For this review, take the finished solid that the model builds, in its own axes (mm). Coordinates: 2 decimals unless noted, no trailing zeros. Write each loop counter-clockwise with the first axis right and the second up, starting at its lowest first coordinate (ties: lowest second). Pieces come first, ordered by that corner, then holes.
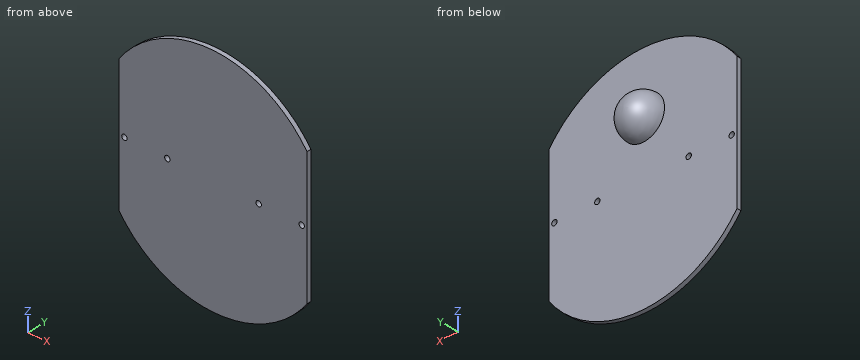
Autodesk Inventor part; units mm, degrees
ref_plane "YZ Plane" through (0, 0, 0) normal (1, 0, 0) x (0, 1, 0)
ref_plane "XZ Plane" through (0, 0, 0) normal (0, 1, 0) x (-1, 0, 0)
ref_plane "XY Plane" through (0, 0, 0) normal (0, 0, 1) x (1, 0, 0)
sketch "Sketch1" plane through (0, 0, 0) normal (0, 1, 0) x (-1, 0, 0)
  line L0 (44.45, 31.7246) -> (44.45, -31.7246)
  line L1 (-44.45, -31.7246) -> (-44.45, 31.7246)
  arc A0 (-44.45, -31.7246) -> (44.45, -31.7246) centre (0, 0) ccw
  arc A1 (44.45, 31.7246) -> (-44.45, 31.7246) centre (0, 0) ccw
  line L2 (44.45, 0) -> (41.91, 0)
  circle A2 centre (41.91, 0) radius 1.27
  line L3 (41.91, 0) -> (21.59, 0)
  circle A3 centre (21.59, 0) radius 1.27
  line L4 (0, -54.61) -> (0, 54.61)
  circle A4 centre (-41.91, 0) radius 1.27
  circle A5 centre (-21.59, 0) radius 1.27
  dimension "d3" = 88.9
  dimension "d4" = 2.54
  dimension "d5" = 2.54
  dimension "d6" = 20.32
  dimension "d7" = 2.54
extrude "Extrusion1" add sketch "Sketch1" along normal blind 2.032
sketch "Sketch2" plane through (0, 2.032, 0) normal (0, 1, 0) x (1, 0, 0)
  circle A0 centre (0, -25.3797) radius 10.16
  point P0 (0, 0)
  dimension "d10" = 20.32
extrude "Extrusion2" add sketch "Sketch2" along normal blind 10.16
fillet "Fillet1" radius 10.16 1 edges at (-10.16, 12.192, 25.3797)
properties part number "Base Plate"
1) Clearance check with flat-ended pins moving along their axes: P1, Ø2, axis at x = -18, y = 2.5, coming from the +Z side; P2, Ø12, axis at x = 31.5, z = -33, coming from the -Y side; P3, Ø12, axis at x = -9, z = -1, coming from the +Y side. State where each tip first meets the part, or that it passes through.
2) Consider section A-A (z = 0). Give the boundary of the cut face in (x, y), then the cut area to 3 significant figures.
3) Consider section D-D (x = 41.91). Give the boundary of the cut face in (y, z), then the cut area to 3 significant figures.
4) Consider section B-B (x = 21.59). Give the boundary of the cut face in (y, z).
5) For L1, parallel to Y at x = -24, z = -29; L2, parallel to Z at x = -41.91, y = 0.8; L3, parallel to Z at x = -21.59, y = 0.85, list the stretches that pass through material, from the lowest coordinate up.
6) Consider section C-C (z = -18). Give the boundary of the cut face in (x, y).
Results:
1. P1: stops at z = 51.86
1. P2: stops at y = 0
1. P3: stops at y = 2.03
2. outline: (-44.45, 0) - (-43.18, 0) - (-43.18, 2.03) - (-44.45, 2.03) - close; (-40.64, 0) - (-22.86, 0) - (-22.86, 2.03) - (-40.64, 2.03) - close; (-20.32, 0) - (20.32, 0) - (20.32, 2.03) - (-20.32, 2.03) - close; (22.86, 0) - (40.64, 0) - (40.64, 2.03) - (22.86, 2.03) - close; (43.18, 0) - (44.45, 0) - (44.45, 2.03) - (43.18, 2.03) - close
2. area: 160 mm2
3. outline: (0, -35.01) - (2.03, -35.01) - (2.03, -1.27) - (0, -1.27) - close; (0, 1.27) - (2.03, 1.27) - (2.03, 35.01) - (0, 35.01) - close
3. area: 137 mm2
4. outline: (0, -50.16) - (2.03, -50.16) - (2.03, -1.27) - (0, -1.27) - close; (0, 1.27) - (2.03, 1.27) - (2.03, 50.16) - (0, 50.16) - close
5. L1: y = 0 to 2.03
5. L2: z = -35.01 to -1.27, 1.27 to 35.01
5. L3: z = -50.16 to -1.27, 1.27 to 50.16
6. outline: (-44.45, 0) - (44.45, 0) - (44.45, 2.03) - (-44.45, 2.03) - close
